from build123d import *

# Parameters (mm, degrees)
BOSS_EXTRUDE1_DEPTH      = 3
BOSS_EXTRUDE1_DEPTH_BACK = 3
SKETCH2_R                = 8
CUT_EXTRUDE1_DEPTH       = 1
CUT_EXTRUDE1_DEPTH_BACK  = 7
SKETCH3_R                = 1.5
CUT_EXTRUDE2_DEPTH       = 1
CUT_EXTRUDE2_DEPTH_BACK  = 7


with BuildPart() as part:
    # Sketch1 → Boss-Extrude1 (new body, two sides)
    with BuildSketch(Plane.XY) as boss_extrude1_sk:
        Polygon((-90, -1414.000005922), (-90, -1359.000005922), (90, -1359.000005922), (90, -1414.000005922), (100, -1414.000005922), (100, -1419.000005922), (70, -1449.000005922), (-70, -1449.000005922), (-100, -1419.000005922), (-100, -1414.000005922), align=None)
    extrude(amount=BOSS_EXTRUDE1_DEPTH)
    extrude(boss_extrude1_sk.sketch, amount=-BOSS_EXTRUDE1_DEPTH_BACK)

    # Sketch2 → Cut-Extrude1 (cut, two sides)
    with BuildSketch(Plane.XY.offset(3)) as cut_extrude1_sk:
        with Locations((0, -1389.000005922)):
            Circle(SKETCH2_R)
    extrude(amount=CUT_EXTRUDE1_DEPTH, mode=Mode.SUBTRACT)
    extrude(cut_extrude1_sk.sketch, amount=-CUT_EXTRUDE1_DEPTH_BACK, mode=Mode.SUBTRACT)

    # Sketch3 → Cut-Extrude2 (cut, two sides)
    with BuildSketch(Plane.XY.offset(3)) as cut_extrude2_sk:
        with Locations((-90, -1414.000005922)):
            Circle(SKETCH3_R)
        with Locations((90, -1414.000005922)):
            Circle(SKETCH3_R)
    extrude(amount=CUT_EXTRUDE2_DEPTH, mode=Mode.SUBTRACT)
    extrude(cut_extrude2_sk.sketch, amount=-CUT_EXTRUDE2_DEPTH_BACK, mode=Mode.SUBTRACT)


solid = part.part
Here's how the part is built. I have some questions about the finished solid (model axes, mm). A direction names the side the tool comes from. Coordinates: 2 decimals unless noted, no trailing zeros. Loops run counter-clockwise (first coordinate to the right, second up) from the corner with the lowest first, then second, coordinate; pieces in that order, holes last.
1. Imagine slicing it at C-C, the plane y = -1391.5. Please give me the cut outline in (x, z), and give its area (3 significant figures).
2. If we mould it in two halves opening along X, with no side actions, what happens to faces 4 (the flat face through (-100, -1417, 0)), 5 (the flat face through (1, -1403, -3)), 6 (the cylindrical face through (-6.349, -1393.868, 0.042)), 7 (the flat face through (90, -1385, 0))? For each: pulls with the +X half, pulls with the -X half, needs draft (parallel to the pull), parting line crosses it, or undercut.
3. Imagine slicing it at D-D, the plane y = -1408.5. Please give me the cut outline in (x, z), and give its area (3 significant figures).
4. For faces 1 (the flat face through (-90, -1386, 0)), 2 (the flat face through (-85, -1434, 0)), 3 (the flat face through (96, -1414, 0)), which set-ups out of +Z, -Z, +X, -X, +Y, -Y let a thin tool reach every point of the face, with its end or its side?
5. Imagine slicing it at B-B, the plane x = 0. Please give me the cut outline in (y, z), and give its area (3 significant figures).
6. Imagine slicing it at A-A, the plane z = -0.85. Please give me the cut outline in (x, y).
7. For P1, Ø3, axis at x = 94, z = -0.5, coming from the +Y side; P2, Ø2, axis at y = -1393, z = 2.5, coming from the -X side; P3, Ø3, axis at y = -1389, z = 0, coming from the +X side, each with a flat end and sliding along its axis, tell me the tip position at first contact or that it passes through.
8. I need wall thicknesses on L1, parallel to Y at x = 0, z = 1.75; L2, parallel to X at y = -1366, z = 2.7; L3, parallel to X at y = -1395, z = -2.4. Which ranges of each line are inside material? Lowest first, please.
Taken from the geometry:
1. outline: (-90, -3) - (-7.6, -3) - (-7.6, 3) - (-90, 3) - close; (7.6, -3) - (90, -3) - (90, 3) - (7.6, 3) - close
1. area: 989 mm2
2. face 4: pulls with the -X half
2. face 5: needs draft
2. face 6: undercut
2. face 7: pulls with the +X half
3. outline: (-90, -3) - (90, -3) - (90, 3) - (-90, 3) - close
3. area: 1,080 mm2
4. face 1: +Z, -Z, -X, +Y
4. face 2: +Z, -Z, -X, -Y
4. face 3: +Z, -Z, +X, +Y
5. outline: (-1449, -3) - (-1397, -3) - (-1397, 3) - (-1449, 3) - close; (-1381, -3) - (-1359, -3) - (-1359, 3) - (-1381, 3) - close
5. area: 444 mm2
6. outline: (-100, -1419) - (-70, -1449) - (70, -1449) - (100, -1419) - (100, -1414) - (91.5, -1414) arc R1.5 cw (long way) to (90, -1412.5) - (90, -1359) - (-90, -1359) - (-90, -1412.5) arc R1.5 cw (long way) to (-91.5, -1414) - (-100, -1414) - close; hole circle Ø16 at (0, -1389)
7. P1: stops at y = -1414
7. P2: stops at x = -90
7. P3: stops at x = 90
8. L1: y = -1449 to -1397, -1381 to -1359
8. L2: x = -90 to 90
8. L3: x = -90 to -5.29, 5.29 to 90
